Build history of the part. All positions in model axes, mm. A direction names the side the tool comes from. Round coordinates to 2 decimals unless told otherwise and drop trailing zeros. Order: outer loops, then holes, each group sorted by start corner. A loop starts at its lowest first (then second) coordinate and runs counter-clockwise, first axis right, second up. Notation, with made-up numbers: (78.5, 26.5) - (90.5, 26.5) arc R7 cw to (90.5, 31.5) - close; hole circle Ø11 at (-29, -1). An arc over 180 degrees is marked (long way). One line per question, with ' | ' between items. Start each with the question number.
from build123d import *

# Parameters (mm, degrees)
ESQUISSE1_R             = 3
BASE_EXTRUSION_DEPTH    = 8
ESQUISSE2_R             = 6
BOSS_EXTRU_1_DEPTH      = 117
ESQUISSE3_R             = 10
BOSS_EXTRU_2_DEPTH      = 17.5
ESQUISSE4_R             = 1.5
ENL_V_MAT_EXTRU_1_DEPTH = 35


with BuildPart() as part:
    # Esquisse1 → Base-Extrusion (new body)
    with BuildSketch(Plane.XY):
        Polygon((0, 6), (0, -6), (70, -30), (95, -30), (95, -20), (70, -20), (25, 0), (70, 20), (95, 20), (95, 30), (70, 30), align=None)
        with Locations((10, 0)):
            Circle(ESQUISSE1_R, mode=Mode.SUBTRACT)
    extrude(amount=BASE_EXTRUSION_DEPTH)

    # Esquisse2 → Boss.-Extru.1 (add)
    with BuildSketch(Plane.ZY):
        with Locations(Location((0, 0, 0), (0, 0, 90))):
            Circle(ESQUISSE2_R)
    extrude(amount=BOSS_EXTRU_1_DEPTH)

    # Esquisse3 → Boss.-Extru.2 (add, symmetric)
    with BuildSketch(Plane(origin=(0, 0, 0), x_dir=(1, 0, 0), z_dir=(0, 1, 0))):
        with Locations(Location((-107, 0, 0), (0, 0, 270))):
            Circle(ESQUISSE3_R)
    extrude(amount=BOSS_EXTRU_2_DEPTH, both=True)

    # Esquisse4 → Enlèv. mat.-Extru.1 (cut)
    with BuildSketch(Plane(origin=(0, 17.5, 0), x_dir=(-1, 0, 0), z_dir=(0, 1, 0))):
        with Locations(Location((107, 0, 0), (0, 0, 90))):
            Circle(ESQUISSE4_R)
    extrude(amount=-ENL_V_MAT_EXTRU_1_DEPTH, mode=Mode.SUBTRACT)


solid = part.part
Item 1: Pin check, flat tips, straight feed: pin 1 (10 mm diameter, centred on x = -108, z = -2, fed in from -Y); pin 2 (7 mm diameter, centred on x = 10, y = 0, fed in from -Z); pin 3 (6 mm diameter, centred on x = -106, z = -2, fed in from +Y). Stop position of each tip, or through.
Item 2: Slice it at B-B (y = 23.5). Write the cut outline in (x, z), plus the area to 3 significant figures.
Item 3: Wall check: line 1 along Y through (x, z) = (10, 5.75); line 2 along Z through (x, y) = (28.5, 8.5); line 3 along X through (y, z) = (8.5, 8.25). Give the ranges that are in metal, low to high. Write a range as [from, to].
Item 4: Slice it at C-C (x = 10). Write the cut outline in (y, z).
Item 5: Pull direction Y, two halves, no side cores. Call faces 6 (the face through (82, 20, 4)), 7 (the face through (-100.24, 0.25, -7.37)), 8 (the face through (35, 18, 4)): released by +Y, released by -Y, zero draft, split by the parting line, or undercut.
Item 6: 3-axis set-ups, long thin cutter, end or side, ignore diameter. For faces 1 (the face through (-107, 17.5, 2)), 2 (the face through (0, 0, -2)), 3 (the face through (-48.807, 5.723, -1.802)), 4 (the face through (-116, 0, -6)), 5 (the face through (83, -20, 4)): which of +Z, -Z, +X, -X, +Y, -Y reach the whole face in a straight line?
Item 7: Slice it at A-A (x = 50.5). Write the cut outline in (y, z).
A:
1) pin 1: y = -17.5 | pin 2: z = 0 | pin 3: y = 17.5
2) outline: (51.04, 0) - (95, 0) - (95, 8) - (51.04, 8) - close | area: 352 mm^2
3) line 1: [-9.43, -3], [3, 9.43] | line 2: [0, 8] | line 3: [-112.65, -101.35]
4) outline: (-9.43, 0) - (-3, 0) - (-3, 8) - (-9.43, 8) - close; (3, 0) - (9.43, 0) - (9.43, 8) - (3, 8) - close
5) face 6: undercut | face 7: zero draft | face 8: released by +Y
6) face 1: +Z, -Z, -X, +Y | face 2: -Z, +X, +Y, -Y | face 3: none | face 4: -Z, -X | face 5: +Z, -Z, +X
7) outline: (-23.31, 0) - (-11.33, 0) - (-11.33, 8) - (-23.31, 8) - close; (11.33, 0) - (23.31, 0) - (23.31, 8) - (11.33, 8) - close
